from build123d import *

# Parameters (mm, degrees)
MODEL_R             = 1.6
EXTRUDE_1_DEPTH     = 4
CUT_EXTRUDE_START   = -3
SKETCH_2_R          = 2.8
SKETCH_2_R_2        = 1.6
CUT_EXTRUDE_1_DEPTH = 3
EXTRUDE_2_DEPTH     = 29
SKETCH_6_R          = 0.725
CUT_EXTRUDE_2_DEPTH = 7


with BuildPart() as part:
    # Model → 凸台-拉伸1 (new body)
    with BuildSketch(Plane.XY):
        Polygon((257.555719115, 185.180286748), (276.055719115, 185.180286748), (276.055719115, 187.180286748), (280.055719115, 187.180286748), (280.055719115, 185.180286748), (320.055719115, 185.180286748), (320.055719115, 187.180286748), (324.055719115, 187.180286748), (324.055719115, 185.180286748), (364.055719115, 185.180286748), (364.055719115, 187.180286748), (368.055719115, 187.180286748), (368.055719115, 185.180286748), (386.555719115, 185.180286748), (386.555719115, 173.180286748), (388.555719115, 173.180286748), (388.555719115, 169.180286748), (386.555719115, 169.180286748), (386.555719115, 137.180286748), (388.555719115, 137.180286748), (388.555719115, 133.180286748), (386.555719115, 133.180286748), (386.555719115, 121.180286748), (368.055719115, 121.180286748), (368.055719115, 119.180286748), (364.055719115, 119.180286748), (364.055719115, 121.180286748), (332.555719115, 121.180286748), (332.555719115, 182.680286748), (311.555719115, 182.680286748), (311.555719115, 121.180286748), (280.055719115, 121.180286748), (280.055719115, 119.180286748), (276.055719115, 119.180286748), (276.055719115, 121.180286748), (257.555719115, 121.180286748), (257.555719115, 133.180286748), (255.555719115, 133.180286748), (255.555719115, 137.180286748), (257.555719115, 137.180286748), (257.555719115, 169.180286748), (255.555719115, 169.180286748), (255.555719115, 173.180286748), (257.555719115, 173.180286748), align=None)
        with Locations((342.055719115, 153.180286748)):
            Circle(MODEL_R, mode=Mode.SUBTRACT)
        with Locations((302.055719115, 153.180286748)):
            Circle(MODEL_R, mode=Mode.SUBTRACT)
    extrude(amount=EXTRUDE_1_DEPTH)

    # 草图2 → 切除-拉伸1 (cut)
    # profile 1 of 2: a face of its own
    with BuildSketch(Plane.XY.offset(4).offset(CUT_EXTRUDE_START)):
        with Locations((302.055719115, 153.180286748)):
            Circle(SKETCH_2_R)
        with Locations((302.055719115, 153.180286748)):
            Circle(SKETCH_2_R_2, mode=Mode.SUBTRACT)
    # profile 2 of 2: a face of its own
    with BuildSketch(Plane.XY.offset(4).offset(CUT_EXTRUDE_START)):
        with Locations((342.055719115, 153.180286748)):
            Circle(SKETCH_2_R)
        with Locations((342.055719115, 153.180286748)):
            Circle(SKETCH_2_R_2, mode=Mode.SUBTRACT)
    extrude(amount=CUT_EXTRUDE_1_DEPTH, mode=Mode.SUBTRACT)

    # 草图3 → 凸台-拉伸2 (add)
    with BuildSketch(Plane.XY.offset(4)):
        Polygon((260.555719115, 182.680286748), (260.555719115, 124.180286748), (311.555719115, 124.180286748), (311.555719115, 121.180286748), (280.055719115, 121.180286748), (280.055719115, 119.180286748), (276.055719115, 119.180286748), (276.055719115, 121.180286748), (257.555719115, 121.180286748), (257.555719115, 133.180286748), (255.555719115, 133.180286748), (255.555719115, 137.180286748), (257.555719115, 137.180286748), (257.555719115, 169.180286748), (255.555719115, 169.180286748), (255.555719115, 173.180286748), (257.555719115, 173.180286748), (257.555719115, 185.180286748), (276.055719115, 185.180286748), (276.055719115, 187.180286748), (280.055719115, 187.180286748), (280.055719115, 185.180286748), (320.055719115, 185.180286748), (320.055719115, 187.180286748), (324.055719115, 187.180286748), (324.055719115, 185.180286748), (364.055719115, 185.180286748), (364.055719115, 187.180286748), (368.055719115, 187.180286748), (368.055719115, 185.180286748), (386.555719115, 185.180286748), (386.555719115, 173.180286748), (388.555719115, 173.180286748), (388.555719115, 169.180286748), (386.555719115, 169.180286748), (386.555719115, 137.180286748), (388.555719115, 137.180286748), (388.555719115, 133.180286748), (386.555719115, 133.180286748), (386.555719115, 121.180286748), (368.055719115, 121.180286748), (368.055719115, 119.180286748), (364.055719115, 119.180286748), (364.055719115, 121.180286748), (332.555719115, 121.180286748), (332.555719115, 124.180286748), (383.555719115, 124.180286748), (383.555719115, 182.680286748), align=None)
    extrude(amount=EXTRUDE_2_DEPTH)

    # 草图6 → 切除-拉伸2 (cut)
    with BuildSketch(Plane.XY.offset(33)):
        with Locations((259.055719115, 183.680286748)):
            Circle(SKETCH_6_R)
        with Locations((385.055719115, 183.680286748)):
            Circle(SKETCH_6_R)
        with Locations((385.055719115, 122.680286748)):
            Circle(SKETCH_6_R)
        with Locations((259.055719115, 122.680286748)):
            Circle(SKETCH_6_R)
    extrude(amount=-CUT_EXTRUDE_2_DEPTH, mode=Mode.SUBTRACT)


solid = part.part
Work out the finished part from the listing and answer in its coordinate system (mm). A direction names the side the tool comes from. Round coordinates to 2 decimals unless told otherwise and drop trailing zeros. Order: outer loops, then holes, each group sorted by start corner. A loop starts at its lowest first (then second) coordinate and runs counter-clockwise, first axis right, second up. Notation, with made-up numbers: M 56,22.25 L 75,22.25 A16 ccw 75,52.25 Z; hole C -34,63 d8. An arc over 180 degrees is marked long. Put each result on its own line as item: value. Start each with the question number.
Q1. Section A-A, the plane x = 376.5 is taken. Write down the section's boundary in (y, z), and give its area (4 significant figures).
Q2. A tool of negligible diameter and unlimited length cuts with its end or side. For faces 1 (the flat face through (267, 121.18, 16)), 2 (the flat face through (344, 185.18, 16)), 3 (the flat face through (383.556, 153, 18)), 4 (the flat face through (386.556, 179, 16)), 5 (the flat face through (257.556, 153, 16)), from which of +Z, -Z, +X, -X, +Y, -Y can it reach the whole face along a straight path? Write none if from no direction.
Q3. Flat-ended cylindrical pins translate along their axes: pin 1 (12 mm diameter, centred on x = 290.5, y = 163.5, fed in from +Z); pin 2 (10 mm diameter, centred on y = 164, z = 11.5, fed in from -X); pin 3 (1 mm diameter, centred on x = 373, z = 10.5, fed in from +Y). Find the tip coordinate at first contact, or state that the pin passes through.
Q4. Section C-C, the plane z = 28 is taken. Give the number of separate pieces and of enclosed holes in the cut face, and give its area (3 significant figures).
Q5. Straight lines are drawn through the part: L1, parallel to X at y = 164, z = 22; L2, parallel to Y at x = 359.5, z = 31; L3, parallel to Z at x = 297, y = 173. For each, find the intervals that lie inside material, in ascending order. Write a range as [from, to].
Q6. Section B-B, the plane y = 139.5 is taken. Write down the section's boundary in (x, z).
Q7. For a pull along X with two mould halves and no side action, classify faces 6 (the flat face through (311.556, 148, 3)), 7 (the flat face through (257.556, 179, 16)), 8 (the flat face through (366, 119.18, 16)) as pulls with the +X half, pulls with the -X half, needs draft (parallel to the pull), parting line crosses it, or undercut.
Findings below:
1. outline: M 121.18,0 L 185.18,0 L 185.18,33 L 182.68,33 L 182.68,4 L 124.18,4 L 124.18,33 L 121.18,33 Z
1. area: 415.5 mm^2
2. face 1: +Z, -Z, -X, -Y
2. face 2: +Z, -Z, +Y
2. face 3: +Z
2. face 4: +Z, -Z, +X, +Y
2. face 5: +Z, -Z, -X
3. pin 1: stops at z = 4
3. pin 2: stops at x = 257.56
3. pin 3: stops at y = 185.18
4. separate pieces: 1
4. enclosed holes: 4
4. area: 1,060 mm^2
5. L1: x = [257.56, 260.56], [383.56, 386.56]
5. L2: y = [121.18, 124.18], [182.68, 185.18]
5. L3: z = [0, 4]
6. outline: M 257.56,0 L 311.56,0 L 311.56,4 L 260.56,4 L 260.56,33 L 257.56,33 Z; M 332.56,0 L 386.56,0 L 386.56,33 L 383.56,33 L 383.56,4 L 332.56,4 Z
7. face 6: undercut
7. face 7: pulls with the -X half
7. face 8: needs draft
